The listing builds one solid part. Answer for the finished solid, in the listing's coordinates (mm). A direction names the side the tool comes from. Give positions to 0.01 mm unless a question says otherwise; leave off trailing zeros. Write each loop counter-clockwise with the first axis right and the second up, starting at its lowest first coordinate (ties: lowest second). Pieces come first, ordered by that corner, then holes.
```python
from build123d import *

# Parameters (mm, degrees)
SKETCH024_W  = 37
SKETCH024_H  = 22
PAD013_DEPTH = 2
SKETCH025_W  = 37
SKETCH025_H  = 2
PAD014_DEPTH = 38
SKETCH027_W  = 1.75
SKETCH027_H  = 12
PAD015_DEPTH = 5


with BuildPart() as part:
    # Sketch024 → Pad013 (new body)
    with BuildSketch(Plane.XZ.offset(7.3)):
        with Locations((-3.25, -29.610007)):
            Rectangle(SKETCH024_W, SKETCH024_H)
    extrude(amount=PAD013_DEPTH)

    # Sketch025 (on Face5 of Pad013) → Pad014 (join)
    with BuildSketch(Plane(origin=(0, -7.3, 0), x_dir=(1, 0, 0), z_dir=(0, 1, 0))):
        with Locations((-3.25, 28.110007)):
            Rectangle(SKETCH025_W, SKETCH025_H)
    extrude(amount=PAD014_DEPTH)

    # Sketch027 (on Face6 of Pad014) → Pad015 (join)
    with BuildSketch(Plane(origin=(0, 0, -27.110007), x_dir=(-1, 0, 0), z_dir=(0, 0, 1))):
        with Locations((16.475, -1.5)):
            Rectangle(SKETCH027_W, SKETCH027_H)
    extrude(amount=PAD015_DEPTH)


solid = part.part
```
Item 1: A cutting plane is placed at C-C, the plane x = 8.5. Give the vertices of the cut face in (y, z).
Conclusion:
outline: (-9.3, -40.61) - (-7.3, -40.61) - (-7.3, -29.11) - (30.7, -29.11) - (30.7, -27.11) - (-7.3, -27.11) - (-7.3, -18.61) - (-9.3, -18.61) - close
Item 2: A cutting plane is placed at B-B, the plane y = -1. Give the vertices of the cut face in (x, z).
Conclusion:
outline: (-21.75, -29.11) - (15.25, -29.11) - (15.25, -27.11) - (-15.6, -27.11) - (-15.6, -22.11) - (-17.35, -22.11) - (-17.35, -27.11) - (-21.75, -27.11) - close
Item 3: A cutting plane is placed at A-A, the plane z = -26. Give the vertices of the cut face in (x, y), plus the area to 3 significant figures.
Conclusion:
outline: (-21.75, -9.3) - (15.25, -9.3) - (15.25, -7.3) - (-21.75, -7.3) - close; (-17.35, -4.5) - (-15.6, -4.5) - (-15.6, 7.5) - (-17.35, 7.5) - close
area: 95.0 mm2
Item 4: Consider probe 1 along Z at (x, y) = (-12, 5.5); probe 2 along Y at (x, z) = (-4, -34.75). Determine where each line is inside the solid, lowest interval first.
Conclusion:
probe 1: z = -29.11 to -27.11
probe 2: y = -9.3 to -7.3
Item 5: Which of the six approach directions +Z, -Z, +X, -X, +Y, -Y give full straight-line access (tool end or side, diameter ignored) to faces 1 (the face through (-15.6, 2, -25)), 2 (the face through (-16, 7.5, -25)), 3 (the face through (-4, 11, -29.11))?
Conclusion:
face 1: +Z, +X, +Y
face 2: +Z, +X, -X, +Y
face 3: -Z, +X, -X, +Y
Item 6: A cutting plane is placed at D-D, the plane z = -21.5. Give the vertices of the cut face in (x, y).
Conclusion:
outline: (-21.75, -9.3) - (15.25, -9.3) - (15.25, -7.3) - (-21.75, -7.3) - close
Item 7: Each of these flat-tipped pins is pushed along its axis until it touches: P1, Ø1.5, axis at x = -13.5, y = 2, coming from the +Z side; P2, Ø5, axis at y = 14.5, z = -22.5, coming from the -X side; P3, Ø2.5, axis at y = 4, z = -24, coming from the +X side; P4, Ø1.9, axis at x = -16.5, y = 3.5, coming from the +Z side. Where does it stop, or does it pass through?
Conclusion:
P1: stops at z = -27.11
P2: passes through
P3: stops at x = -15.6
P4: stops at z = -22.11
